Design review of the part built by this model. Coordinates are the model's own, in mm. A direction names the side the tool comes from. Give positions to 0.01 mm unless a question says otherwise; leave off trailing zeros. Loops run counter-clockwise (first coordinate to the right, second up) from the corner with the lowest first, then second, coordinate; pieces in that order, holes last. Notation, with made-up numbers: M -3,3 L 18,3 A25 ccw 18,15 Z; hole C 37,79 d11. An arc over 180 degrees is marked long. Use CSV: the item, a comma, the result in double quotes.
from build123d import *

# Parameters (mm, degrees)
SKIZZE4_R                       = 6
SCHNITT_LINEAR_AUSTRAGEN2_DEPTH = 51
VERRUNDUNG2_R                   = 5


with BuildPart() as part:
    # Skizze2 → Rotation2 (revolve)
    with BuildSketch(Plane.XY, mode=Mode.PRIVATE) as rotation2_sk:
        with BuildLine():
            Line((0, 14.040713887), (0, 50))
            Line((0, 50), (-10, 50))
            Line((-10, 50), (-10, 14.040713887))
            ThreePointArc((-10, 14.040713887), (-21.345292125, 8.936630056), (-30, 0))
            Line((-30, 0), (-30, -10))
            Line((-30, -10), (-25.817799793, -10))
            Line((-25.817799793, -10), (-25.817799793, -2.740292215))
            ThreePointArc((-25.817799793, -2.740292215), (-18.472392098, 4.844387952), (-8.843436705, 9.176316562))
            Line((-8.843436705, 9.176316562), (0, 9.176316562))
            Line((0, 9.176316562), (0, 14.040713887))
        make_face()
    revolve(rotation2_sk.sketch.rotate(Axis((0, 14.040713887, 0), (0, 1, 0)), 270), axis=Axis((0, 14.040713887, 0), (0, 1, 0)))  # turned: the seam where the file's is

    # Skizze4 → Schnitt-Linear austragen2 (cut, through all)
    with BuildSketch(Plane(origin=(0, 0, 0), x_dir=(1, 0, 0), z_dir=(0, 1, 0))):
        with Locations(Location((0, 0, 0), (0, 0, 270))):  # turned: the seam where the file's is
            Circle(SKIZZE4_R)
    extrude(amount=SCHNITT_LINEAR_AUSTRAGEN2_DEPTH, mode=Mode.SUBTRACT)

    # Verrundung2
    verrundung2_edges = [part.edges().sort_by_distance(p)[0] for p in [
        (0, 0, 30),
    ]]
    fillet(verrundung2_edges, radius=VERRUNDUNG2_R)


solid = part.part
(1) We need section A-A on y = 19. State the section outline as (x, z) points.
A:
outline,"C 0,0 d20; hole C 0,0 d12"
(2) Machinability: for faces 1 (the cylindrical face through (-25.6, -6.32, 3.36)), 2 (the cylindrical face through (1.802, 29.302, 5.723)), 3 (the cylindrical face through (9.76, 31.77, 2.17)), which of the approach directions +Z, -Z, +X, -X, +Y, -Y give a long, thin tool a straight path to every point of the face, cutting with its end or side? Answer none if there is none.
A:
face 1,"-Y"
face 2,"+Y, -Y"
face 3,"+Y"
(3) The part is to be moulded in two halves that separate along X. For faces 4 (the flat face through (-22.4, -10, -13.2)), 5 (the flat face through (6, 9.176, -2)), 6 (the cylindrical face through (-1.32, -5.84, 29.97)), say which applies: released by +X, released by -X, zero draft, split by the parting line, or undercut.
A:
face 4,"zero draft"
face 5,"undercut"
face 6,"split by the parting line"
(4) Wall thickness on line 1 along X through (y, z) = (-5.25, 0); line 2 along X through (y, z) = (18, 0); line 3 along Z through (x, y) = (-5.5, 3): over which ranges is each line inside the solid? List them lowest first. Write a range as [from, to].
A:
line 1,"[-30, -25.82], [25.82, 30]"
line 2,"[-10, -6], [6, 10]"
line 3,"[-27.23, -20.08], [20.08, 27.23]"
(5) Clearance check with flat-ended pins moving along their axes: P1, Ø5, axis at y = 24, z = -2.5, coming from the -X side; P2, Ø6, axis at x = 5.5, y = 4, coming from the +Z side; P3, Ø2, axis at y = 3, z = -17.5, coming from the +X side; P4, Ø11, axis at x = 0, z = 0, coming from the +Y side. State where each tip first meets the part, or that it passes through.
A:
P1,"x = -10"
P2,"z = 28.85"
P3,"x = 22.86"
P4,"through"
